Design review of the part shown in the three views and the two pictorial views. Dimensions are in mm from the part's minimum x, y and z. A direction names the side the tool comes from. Coordinates: 2 decimals unless noted, no trailing zeros. Loops run counter-clockwise (first coordinate to the right, second up) from the corner with the lowest first, then second, coordinate; pieces in that order, holes last. Notation, with made-up numbers: (-29.75, 44.5) -> (-7.75, 44.5) arc R3 ccw to (-7.75, 49.5) -> close; hole circle Ø6 at (3, 38). An arc over 180 degrees is marked (long way). Answer in a Markdown table with one row per item.
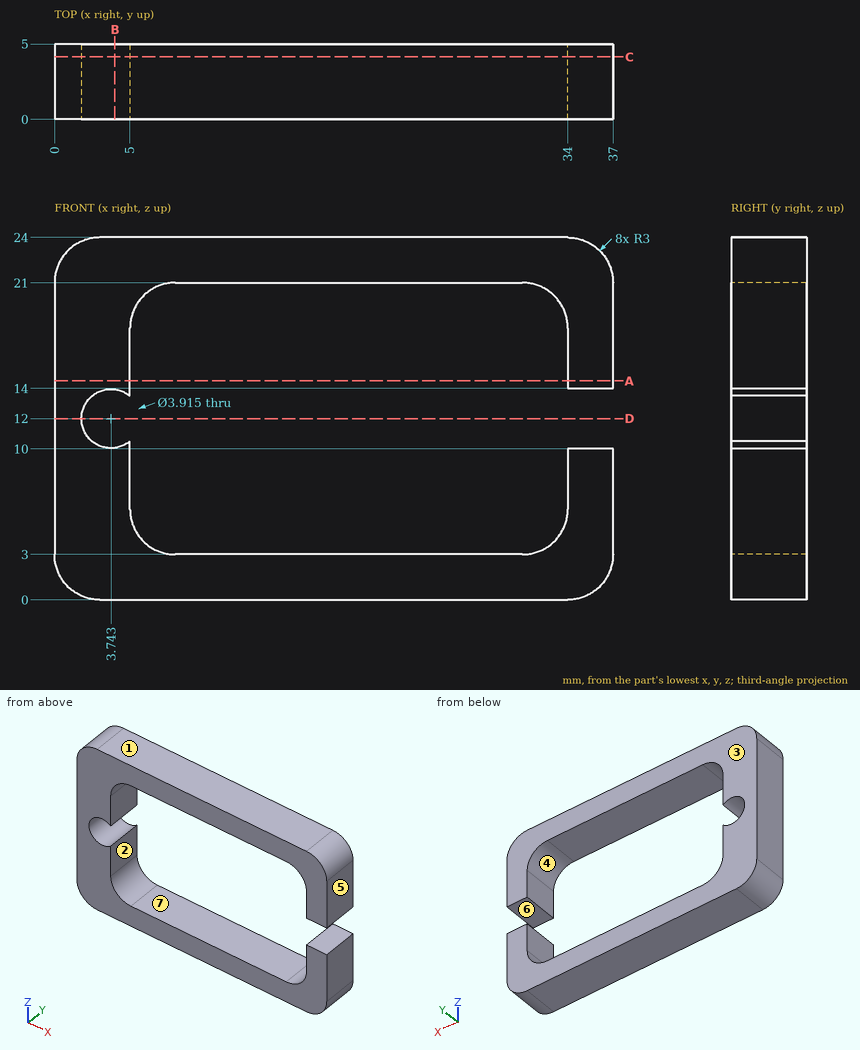
(1) Take a section at A-A on z = 14.5. Give the boundary of the cut face in (x, y), and give its area (3 significant figures).
Evaluation:
| item | result |
|---|---|
| outline | (0, 0) -> (5, 0) -> (5, 5) -> (0, 5) -> close; (34, 0) -> (37, 0) -> (37, 5) -> (34, 5) -> close |
| area | 40.0 mm² |
(2) Take a section at B-B on x = 4. Give the boundary of the cut face in (y, z).
Evaluation:
| item | result |
|---|---|
| outline | (0, 0) -> (5, 0) -> (5, 10.06) -> (0, 10.06) -> close; (0, 13.94) -> (5, 13.94) -> (5, 24) -> (0, 24) -> close |
(3) To check wall thickness, follow probe 1 along Z at (x, y) = (14, 3.45); probe 2 along X at (y, z) = (1.9, 19.5); probe 3 along X at (y, z) = (1.25, 12) (1 decimal). State the ranges of each line that lie inside material, in increasing order.
Evaluation:
| item | result |
|---|---|
| probe 1 | z = 0 to 3, 21 to 24 |
| probe 2 | x = 0 to 5.4, 33.6 to 37 |
| probe 3 | x = 0 to 1.8 |
(4) For pin 1 (2 mm diameter, centred on y = 3.5, z = 8.5, fed in from -X); pin 2 (1.5 mm diameter, centred on x = 36, y = 1.5, fed in from -Z), all flat-tipped, find the tip position at first contact; note any pin that passes through.
Evaluation:
| item | result |
|---|---|
| pin 1 | stops at x = 0 |
| pin 2 | stops at z = 0.27 |
(5) Take a section at D-D on z = 12. Give the boundary of the cut face in (x, y) (1 decimal).
Evaluation:
| item | result |
|---|---|
| outline | (0, 0) -> (1.8, 0) -> (1.8, 5) -> (0, 5) -> close |
(6) Draft analysis for pull direction Z (two halves, no side actions). For the marked faces 1, 2, 3 and 4, state which applies: pulls with the +Z half, pulls with the -Z half, needs draft (parallel to the pull), parting line crosses it, or undercut.
Evaluation:
| item | result |
|---|---|
| face 1 | pulls with the +Z half |
| face 2 | undercut |
| face 3 | needs draft |
| face 4 | undercut |
(7) Take a section at C-C on y = 4.15. Give the boundary of the cut face in (x, z) (1 decimal).
Evaluation:
| item | result |
|---|---|
| outline | (0, 3) arc R3 ccw to (3, 0) -> (34, 0) arc R3 ccw to (37, 3) -> (37, 10) -> (34, 10) -> (34, 6) arc R3 cw to (31, 3) -> (8, 3) arc R3 cw to (5, 6) -> (5, 10.5) arc R2 cw (long way) to (5, 13.5) -> (5, 18) arc R3 cw to (8, 21) -> (31, 21) arc R3 cw to (34, 18) -> (34, 14) -> (37, 14) -> (37, 21) arc R3 ccw to (34, 24) -> (3, 24) arc R3 ccw to (0, 21) -> close |
(8) Tool access review of the marked faces 5, 6 and 7: name each direction out of +Z, -Z, +X, -X, +Y, -Y from which nothing blocks a thin tool from reaching the whole face with its end or side.
Evaluation:
| item | result |
|---|---|
| face 5 | +Z, -Z, +X, +Y, -Y |
| face 6 | +X, +Y, -Y |
| face 7 | +Y, -Y |
